Work out the finished part from the listing and answer in its coordinate system (mm). A direction names the side the tool comes from. Round coordinates to 2 decimals unless told otherwise and drop trailing zeros. Write each loop counter-clockwise with the first axis right and the second up, starting at its lowest first coordinate (ties: lowest second). Pieces come first, ordered by that corner, then holes. Notation, with made-up numbers: (74.5, -1.5) -> (104.5, -1.5) arc R24 cw to (104.5, 9.5) -> close; hole circle Ø1 at (83, -23.5). An arc over 180 degrees is marked (long way). One line per question, with ' | ' between items. Start each with the question number.
```python
from build123d import *

# Parameters (mm, degrees)
SKETCH1_W           = 5.5
SKETCH1_H           = 6.1
SKETCH1_W_2         = 3.3
SKETCH1_H_2         = 3.3
BOSS_EXTRUDE1_DEPTH = 7
SKETCH2_W           = 5.5
SKETCH2_H           = 6.1
BOSS_EXTRUDE2_DEPTH = 1.5
SKETCH3_W           = 7
SKETCH3_H           = 12.1
SKETCH3_W_2         = 3.3
SKETCH3_H_2         = 3.3
BOSS_EXTRUDE3_DEPTH = 1.5
FILLET1_R           = 1


with BuildPart() as part:
    # Sketch1 → Boss-Extrude1 (new body)
    with BuildSketch(Plane(origin=(0, 0, 0), x_dir=(1, 0, 0), z_dir=(0, 1, 0))):
        with Locations((2.75, 3.05)):
            Rectangle(SKETCH1_W, SKETCH1_H)
        with Locations((2.85, 3.05)):
            Rectangle(SKETCH1_W_2, SKETCH1_H_2, mode=Mode.SUBTRACT)
    extrude(amount=BOSS_EXTRUDE1_DEPTH)

    # Sketch2 → Boss-Extrude2 (add)
    with BuildSketch(Plane(origin=(0, 7, 0), x_dir=(1, 0, 0), z_dir=(0, 1, 0))):
        with Locations((2.75, 3.05)):
            Rectangle(SKETCH2_W, SKETCH2_H)
    extrude(amount=-BOSS_EXTRUDE2_DEPTH)

    # Sketch3 → Boss-Extrude3 (add)
    with BuildSketch(Plane(origin=(0, 0, 0), x_dir=(1, 0, 0), z_dir=(0, 1, 0))):
        with Locations((2, 3.05)):
            Rectangle(SKETCH3_W, SKETCH3_H)
        with Locations((2.85, 3.05)):
            Rectangle(SKETCH3_W_2, SKETCH3_H_2, mode=Mode.SUBTRACT)
    extrude(amount=BOSS_EXTRUDE3_DEPTH)

    # Fillet1
    fillet1_edges = [part.edges().sort_by_distance(p)[0] for p in [
        (5.5, 7, -3.05),
        (2.75, 7, -6.1),
        (0, 7, -3.05),
        (0, 4.25, -6.1),
        (5.5, 4.25, -6.1),
        (5.5, 4.25, 0),
        (0, 4.25, 0),
        (2.75, 7, 0),
    ]]
    fillet(fillet1_edges, radius=FILLET1_R)


solid = part.part
```
(1) Given pin 1 Ø1 at (x, z) = (2, -7.5) entering from +Y; pin 2 Ø1.8 at (x, y) = (3.5, 4.5) entering from -Z; pin 3 Ø4 at (y, z) = (4, -7.5) entering from -X, each flat-ended and moving along its own axis, determine where each tip first touches the part or whether it passes through.
(2) For faces 5 (the flat face through (3, 5.5, -3)), 6 (the cylindrical face through (0.301, 3.782, -0.285)), 7 (the cylindrical face through (5.199, 3.782, -0.285)), determine the directions among +Z, -Z, +X, -X, +Y, -Y from which every point of the face is accessible in a straight line to the end or side of a thin tool.
(3) A cutting plane is placed at A-A, the plane y = 3. Determine the outline of the cut face in (x, z), then the cut area to 3 significant figures.
(4) A cutting plane is placed at D-D, the plane y = 1.25. Determine the outline of the cut face in (x, z).
(5) The mould has two halves that part along Z. Classify faces 1 (the flat face through (3, 3, -4.7)), 2 (the flat face through (3, 3, -1.4)), 3 (the flat face through (-1.5, 1, -3)), 4 (the flat face through (2, 1, 3)): +Z half, -Z half, draft (parallel to the pull), parting line (faces both ways), or undercut.
(6) A cutting plane is placed at B-B, the plane x = 3. Determine the outline of the cut face in (y, z).
(7) A cutting plane is placed at C-C, the plane z = -2. Determine the outline of the cut face in (x, y), then the cut area to 3 significant figures.
(8) Consider L1, parallel to X at y = 4.25, z = -1.75; L2, parallel to Z at x = 1.25, y = 4.75; L3, parallel to Y at x = 4.25, z = 1.25. Determine where each line is inside the solid, lowest interval first.
Returned:
1) pin 1: y = 1.5 | pin 2: z = -6.1 | pin 3: x = 0.08
2) face 5: -Y | face 6: +Z, -X, +Y | face 7: +Z, +X, +Y
3) outline: (0, -5.1) arc R1 ccw to (1, -6.1) -> (4.5, -6.1) arc R1 ccw to (5.5, -5.1) -> (5.5, -1) arc R1 ccw to (4.5, 0) -> (1, 0) arc R1 ccw to (0, -1) -> close; hole (1.2, -4.7) -> (4.5, -4.7) -> (4.5, -1.4) -> (1.2, -1.4) -> close | area: 21.8 mm2
4) outline: (-1.5, -9.1) -> (5.5, -9.1) -> (5.5, 3) -> (-1.5, 3) -> close; hole (1.2, -4.7) -> (4.5, -4.7) -> (4.5, -1.4) -> (1.2, -1.4) -> close
5) face 1: undercut | face 2: undercut | face 3: draft | face 4: +Z half
6) outline: (0, -9.1) -> (1.5, -9.1) -> (1.5, -6.1) -> (6, -6.1) arc R1 ccw to (7, -5.1) -> (7, -1) arc R1 ccw to (6, 0) -> (1.5, 0) -> (1.5, 3) -> (0, 3) -> (0, -1.4) -> (5.5, -1.4) -> (5.5, -4.7) -> (0, -4.7) -> close
7) outline: (-1.5, 0) -> (1.2, 0) -> (1.2, 5.5) -> (4.5, 5.5) -> (4.5, 0) -> (5.5, 0) -> (5.5, 6) arc R1 ccw to (4.5, 7) -> (1, 7) arc R1 ccw to (0, 6) -> (0, 1.5) -> (-1.5, 1.5) -> close | area: 22.2 mm2
8) L1: 0 to 1.2, 4.5 to 5.5 | L2: -6.1 to -4.7, -1.4 to 0 | L3: 0 to 1.5
